```python
from build123d import *

# Parameters (mm, degrees)
SKETCH_1_W             = 60
SKETCH_1_H             = 60
EXTRUDE_1_DEPTH        = 12
HOLE_WIZARD_M121_D     = 10.2
HOLE_WIZARD_M121_DEPTH = 12
SKETCH_12_R            = 4.5
CUT_EXTRUDE_1_DEPTH    = 13
SKETCH_13_R            = 7.5
CUT_EXTRUDE_2_DEPTH    = 9


with BuildPart() as part:
    # Эскиз1 → Бобышка-Вытянуть1 (new body)
    with BuildSketch(Plane(origin=(0, 0, 0), x_dir=(1, 0, 0), z_dir=(0, 1, 0))):
        Rectangle(SKETCH_1_W, SKETCH_1_H)
    extrude(amount=EXTRUDE_1_DEPTH)

    # Отверстие обработанное метчиком M121
    with Locations(Plane(origin=(0, 12, 0), x_dir=(1, 0, 0), z_dir=(0, 1, 0))):
        with Locations((0, 0)):
            Hole(HOLE_WIZARD_M121_D / 2, depth=HOLE_WIZARD_M121_DEPTH)

    # Эскиз12 → Вырез-Вытянуть1 (cut, through all)
    with BuildSketch(Plane(origin=(0, 12, 0), x_dir=(1, 0, 0), z_dir=(0, 1, 0))):
        with Locations(Location((-15, 15, 0), (0, 0, 270))):  # turned: the seam where the file's is
            Circle(SKETCH_12_R)
        with Locations(Location((15, 15, 0), (0, 0, 270))):  # turned: the seam where the file's is
            Circle(SKETCH_12_R)
        with Locations(Location((15, -15, 0), (0, 0, 270))):  # turned: the seam where the file's is
            Circle(SKETCH_12_R)
        with Locations(Location((-15, -15, 0), (0, 0, 270))):  # turned: the seam where the file's is
            Circle(SKETCH_12_R)
    extrude(amount=-CUT_EXTRUDE_1_DEPTH, mode=Mode.SUBTRACT)

    # Эскиз13 → Вырез-Вытянуть2 (cut)
    with BuildSketch(Plane(origin=(0, 12, 0), x_dir=(1, 0, 0), z_dir=(0, 1, 0))):
        with Locations(Location((-15, 15, 0), (0, 0, 270))):  # turned: the seam where the file's is
            Circle(SKETCH_13_R)
        with Locations(Location((15, 15, 0), (0, 0, 270))):  # turned: the seam where the file's is
            Circle(SKETCH_13_R)
        with Locations(Location((15, -15, 0), (0, 0, 270))):  # turned: the seam where the file's is
            Circle(SKETCH_13_R)
        with Locations(Location((-15, -15, 0), (0, 0, 270))):  # turned: the seam where the file's is
            Circle(SKETCH_13_R)
    extrude(amount=-CUT_EXTRUDE_2_DEPTH, mode=Mode.SUBTRACT)


solid = part.part
```
Could you check a few things on this model? Use its own coordinates, in mm. A direction names the side the tool comes from. Round coordinates to 2 decimals unless told otherwise and drop trailing zeros. Loops run counter-clockwise (first coordinate to the right, second up) from the corner with the lowest first, then second, coordinate; pieces in that order, holes last. Notation, with made-up numbers: (57, 59) - (81, 59) arc R32 cw to (81, 97) - close; hole circle Ø6 at (-2, -22.75). An arc over 180 degrees is marked (long way). Answer in a Markdown table with one row per item. Add a question column.
(1) If we section it at B-B (x = -15): Please give me the cut outline in (y, z), plus the area to 3 significant figures.
(2) For faces 5 (the face through (0, 6, 30)), 6 (the face through (10, 3, -15)), which set-ups out of +Z, -Z, +X, -X, +Y, -Y let a thin tool reach every point of the face, with its end or its side?
(3) If we section it at D-D (z = 0): Please give me the cut outline in (x, y).
(4) If we section it at C-C (z = -15): Please give me the cut outline in (x, y), plus the area to 3 significant figures.
(5) If we mould it in two halves opening along Z, with no side actions, what happens to faces 1 (the face through (-14.67, 7.563, -22.493)), 2 (the face through (-30, 6, 0)), 3 (the face through (-10.54, 1.52, 14.41)), 4 (the face through (0, 6, -30))? For each: pulls with the +Z half, pulls with the -Z half, needs draft (parallel to the pull), parting line crosses it, or undercut.
(6) If we section it at A-A (x = 0): Please give me the cut outline in (y, z), plus the area to 3 significant figures.
(7) I'm going to push flat-ended pins straight in: pin 1 (7.5 mm diameter, centred on x = 14, z = 15, fed in from +Y); pin 2 (7 mm diameter, centred on x = -15, z = -15, fed in from +Y). Where does each tip first touch, or does it pass through?
(8) I need wall thicknesses on line 1 along X through (y, z) = (1.75, 15); line 2 along X through (y, z) = (5.5, -15); line 3 along Z through (x, y) = (20, 5.5). Which ranges of each line are inside material? Lowest first, please.
Model answer:
| question | item | result |
|---|---|---|
| 1 | outline | (0, -30) - (12, -30) - (12, -22.5) - (3, -22.5) - (3, -19.5) - (0, -19.5) - close; (0, -10.5) - (3, -10.5) - (3, -7.5) - (12, -7.5) - (12, 7.5) - (3, 7.5) - (3, 10.5) - (0, 10.5) - close; (0, 19.5) - (3, 19.5) - (3, 22.5) - (12, 22.5) - (12, 30) - (0, 30) - close |
| 1 | area | 396 mm² |
| 2 | face 5 | +Z, +X, -X, +Y, -Y |
| 2 | face 6 | +Y |
| 3 | outline | (-30, 0) - (-5.1, 0) - (-5.1, 12) - (-30, 12) - close; (5.1, 0) - (30, 0) - (30, 12) - (5.1, 12) - close |
| 4 | outline | (-30, 0) - (-19.5, 0) - (-19.5, 3) - (-22.5, 3) - (-22.5, 12) - (-30, 12) - close; (-10.5, 0) - (10.5, 0) - (10.5, 3) - (7.5, 3) - (7.5, 12) - (-7.5, 12) - (-7.5, 3) - (-10.5, 3) - close; (19.5, 0) - (30, 0) - (30, 12) - (22.5, 12) - (22.5, 3) - (19.5, 3) - close |
| 4 | area | 396 mm² |
| 5 | face 1 | undercut |
| 5 | face 2 | needs draft |
| 5 | face 3 | undercut |
| 5 | face 4 | pulls with the -Z half |
| 6 | outline | (0, -30) - (12, -30) - (12, -5.1) - (0, -5.1) - close; (0, 5.1) - (12, 5.1) - (12, 30) - (0, 30) - close |
| 6 | area | 598 mm² |
| 7 | pin 1 | stops at y = 3 |
| 7 | pin 2 | passes through |
| 8 | line 1 | x = -30 to -19.5, -10.5 to 10.5, 19.5 to 30 |
| 8 | line 2 | x = -30 to -22.5, -7.5 to 7.5, 22.5 to 30 |
| 8 | line 3 | z = -30 to -20.59, -9.41 to 9.41, 20.59 to 30 |
